from build123d import *

# Parameters (mm, degrees)
F1_DEPTH = 1
F2_DEPTH = 10
F3_DEPTH = 700
F5_D     = 4


with BuildPart() as f1:
    # F0 (on Front) → F1 (new body)
    with BuildSketch(Plane.XZ):
        with BuildLine():
            Line((-292.7657316476, 450), (-292.7657316476, -450))
            Line((-292.7657316476, -450), (-287.7657316476, -450))
            Line((-287.7657316476, -450), (-282.7657316476, -450))
            Line((-282.7657316476, -450), (-282.7657316476, 450))
            ThreePointArc((-282.7657316476, 450), (-250.5474775781, 527.7817459305), (-172.7657316476, 560))
            Line((-172.7657316476, 560), (67.2342683524, 560))
            ThreePointArc((67.2342683524, 560), (145.0160142829, 527.7817459305), (177.2342683524, 450))
            Line((177.2342683524, 450), (177.2342683524, -450))
            Line((177.2342683524, -450), (187.2342683524, -450))
            Line((187.2342683524, -450), (187.2342683524, 450))
            ThreePointArc((187.2342683524, 450), (152.0870820948, 534.8528137424), (67.2342683524, 570))
            Line((67.2342683524, 570), (-172.7657316476, 570))
            ThreePointArc((-172.7657316476, 570), (-257.61854539, 534.8528137424), (-292.7657316476, 450))
        make_face()
    extrude(amount=F1_DEPTH)

    # F0 (on Front) → F2 (join)
    with BuildSketch(Plane.XZ):
        with BuildLine():
            Line((-293.2657316476, 450), (-293.2657316476, -450))
            Line((-293.2657316476, -450), (-292.7657316476, -450))
            Line((-292.7657316476, -450), (-292.7657316476, 450))
            ThreePointArc((-292.7657316476, 450), (-257.61854539, 534.8528137424), (-172.7657316476, 570))
            Line((-172.7657316476, 570), (67.2342683524, 570))
            ThreePointArc((67.2342683524, 570), (152.0870820948, 534.8528137424), (187.2342683524, 450))
            Line((187.2342683524, 450), (187.2342683524, -450))
            Line((187.2342683524, -450), (187.7342683524, -450))
            Line((187.7342683524, -450), (187.7342683524, 450))
            ThreePointArc((187.7342683524, 450), (152.4406354854, 535.206367133), (67.2342683524, 570.5))
            Line((67.2342683524, 570.5), (-172.7657316476, 570.5))
            ThreePointArc((-172.7657316476, 570.5), (-257.9720987806, 535.206367133), (-293.2657316476, 450))
        make_face()
        with BuildLine():
            Line((-282.7657316476, 450), (-282.7657316476, -450))
            Line((-282.7657316476, -450), (-282.2657316476, -450))
            Line((-282.2657316476, -450), (-282.2657316476, 450))
            ThreePointArc((-282.2657316476, 450), (-250.1939241875, 527.4281925399), (-172.7657316476, 559.5))
            Line((-172.7657316476, 559.5), (67.2342683524, 559.5))
            ThreePointArc((67.2342683524, 559.5), (144.6624608923, 527.4281925399), (176.7342683524, 450))
            Line((176.7342683524, 450), (176.7342683524, -450))
            Line((176.7342683524, -450), (177.2342683524, -450))
            Line((177.2342683524, -450), (177.2342683524, 450))
            ThreePointArc((177.2342683524, 450), (145.0160142829, 527.7817459305), (67.2342683524, 560))
            Line((67.2342683524, 560), (-172.7657316476, 560))
            ThreePointArc((-172.7657316476, 560), (-250.5474775781, 527.7817459305), (-282.7657316476, 450))
        make_face()
    extrude(amount=F2_DEPTH)

    # F3 (cut): a face of the model
    f3_faces = [f1.faces().sort_by_distance(p)[0] for p in [
        (182.2342683524, -0.1486606875, -450),
    ]]
    extrude(f3_faces, amount=-F3_DEPTH, mode=Mode.SUBTRACT)

    # F5 (through all)
    with Locations(Plane.XZ.offset(1)):
        with Locations((-287.7128323337, 453.4766965134)):
            Hole(F5_D / 2)


solid = f1.part
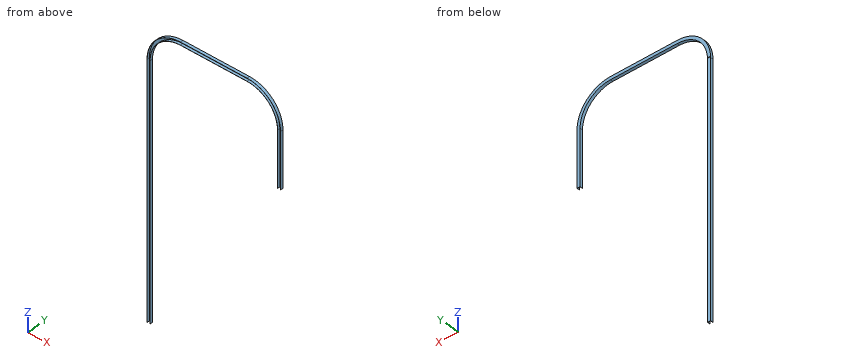
Read the model definition and answer for the solid it produces. Units are mm, in the model's axes. Coordinates: 2 decimals unless noted, no trailing zeros. Loops run counter-clockwise (first coordinate to the right, second up) from the corner with the lowest first, then second, coordinate; pieces in that order, holes last.
Q1. The part is cut by section B-B on z = 357. Write down the section's boundary in (x, y).
Q2. The part is cut by section D-D on z = -312. Write down the section's boundary in (x, y).
Q3. Each of these flat-tipped pins is pushed along its axis until it touches: pin 1 Ø6 at (x, y) = (-138, -3.5) entering from -Z; pin 2 Ø4.5 at (y, z) = (-5.5, 74.5) entering from +X; pin 3 Ø2.5 at (x, z) = (-287.71, 453.48) entering from +Y; pin 4 Ø3 at (x, y) = (-175.5, -6.5) entering from +Z. Where does it stop, or does it pass through?
Q4. The part is cut by section A-A on y = -7.5. Write down the section's boundary in (x, z), and give its area (3 significant figures).
Q5. The part is cut by section C-C on x = -48. Write down the section's boundary in (y, z), and give its area (3 significant figures).
Q6. Consider probe 1 along X at (y, z) = (-2.5, 393.5); probe 2 along X at (y, z) = (-7.5, 137); probe 3 along Z at (x, y) = (6, -3). Determine where each line is inside the solid, lowest interval first.
Results below:
1. outline: (-293.27, -10) - (-292.77, -10) - (-292.77, -1) - (-282.77, -1) - (-282.77, -10) - (-282.27, -10) - (-282.27, 0) - (-293.27, 0) - close; (176.73, -10) - (177.23, -10) - (177.23, -1) - (187.23, -1) - (187.23, -10) - (187.73, -10) - (187.73, 0) - (176.73, 0) - close
2. outline: (-293.27, -10) - (-292.77, -10) - (-292.77, -1) - (-282.77, -1) - (-282.77, -10) - (-282.27, -10) - (-282.27, 0) - (-293.27, 0) - close
3. pin 1: stops at z = 559.5
3. pin 2: stops at x = -282.27
3. pin 3: passes through
3. pin 4: stops at z = 570.49
4. outline: (-293.27, -450) - (-292.77, -450) - (-292.77, 450) arc R120 cw to (-172.77, 570) - (67.23, 570) arc R120 cw to (187.23, 450) - (187.23, 250) - (187.73, 250) - (187.73, 450) arc R120.5 ccw to (67.23, 570.5) - (-172.77, 570.5) arc R120.5 ccw to (-293.27, 450) - close; (-282.77, -450) - (-282.27, -450) - (-282.27, 450) arc R109.5 cw to (-172.77, 559.5) - (67.23, 559.5) arc R109.5 cw to (176.73, 450) - (176.73, 250) - (177.23, 250) - (177.23, 450) arc R110 ccw to (67.23, 560) - (-172.77, 560) arc R110 ccw to (-282.77, 450) - close
4. area: 1,700 mm2
5. outline: (-10, 559.5) - (0, 559.5) - (0, 570.5) - (-10, 570.5) - (-10, 570) - (-1, 570) - (-1, 560) - (-10, 560) - close
5. area: 20.0 mm2
6. probe 1: x = -293.27 to -292.77, -282.77 to -282.27, 176.73 to 177.23, 187.23 to 187.73
6. probe 2: x = -293.27 to -292.77, -282.77 to -282.27
6. probe 3: z = 559.5 to 560, 570 to 570.5
